```python
from build123d import *

# Parameters (mm, degrees)
MOTOR_CLAMP_EXTRUDE_DEPTH = 20
CLAMP_CLEARANCE_HOLE_D    = 3.6
CLAMP_CORNER_FILLETS_R    = 6


with BuildPart() as part:
    # Hold Down Bracket Sketch → Motor Clamp Extrude (new body)
    with BuildSketch(Plane(origin=(0, 0, 0), x_dir=(0, 0, -1), z_dir=(1, 0, 0))):
        with BuildLine():
            Line((-33.5, -23.25), (-29.5, -23.25))
            Line((-29.5, -23.25), (-29.5, -30))
            Line((-29.5, -30), (-25.5, -30))
            Line((-25.5, -30), (-25.5, -19.25))
            Line((-25.5, -19.25), (-33.5, -19.25))
            ThreePointArc((-33.5, -19.25), (-52.75, 0), (-33.5, 19.25))
            Line((-33.5, 19.25), (-25.5, 19.25))
            Line((-25.5, 19.25), (-25.5, 30))
            Line((-25.5, 30), (-29.5, 30))
            Line((-29.5, 30), (-29.5, 23.25))
            Line((-29.5, 23.25), (-33.5, 23.25))
            ThreePointArc((-33.5, 23.25), (-56.75, 0), (-33.5, -23.25))
        make_face()
    extrude(amount=MOTOR_CLAMP_EXTRUDE_DEPTH)

    # Clamp Clearance Hole (through all)
    with Locations(Plane.XY.offset(29.5)):
        with Locations((10, -26.5)):
            clamp_clearance_hole = Hole(CLAMP_CLEARANCE_HOLE_D / 2)

    # Clamp Clearance Hole Mirror: Clamp Clearance Hole across plane
    add(clamp_clearance_hole.mirror(Plane.ZX), mode=Mode.SUBTRACT)

    # Clamp Corner Fillets
    clamp_corner_fillets_edges = [part.edges().sort_by_distance(p)[0] for p in [
        (0, 30, 27.5),
        (0, -30, 27.5),
        (20, -30, 27.5),
        (20, 30, 27.5),
    ]]
    fillet(clamp_corner_fillets_edges, radius=CLAMP_CORNER_FILLETS_R)


solid = part.part
```
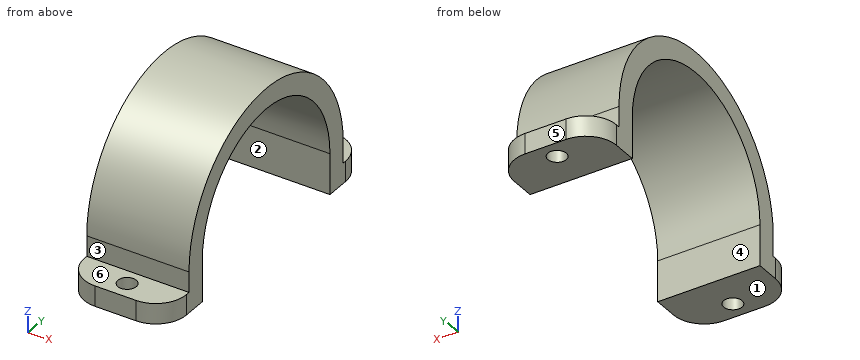
Here's how the part is built. I have some questions about the finished solid (model axes, mm). Face numbers are marked on the shaded views. A direction names the side the tool comes from. Round coordinates to 2 decimals unless told otherwise and drop trailing zeros. Write each loop counter-clockwise with the first axis right and the second up, starting at its lowest first coordinate (ties: lowest second). Pieces come first, ordered by that corner, then holes.
Q1. If we section it at B-B on y = 25.5: Write out the boundary of the cut face in (x, z), plus the area to 3 significant figures.
Q2. Which directions (+Z, -Z, +X, -X, +Y, -Y) give clear straight access to the entire face, cutting with the end or side of a thin tool? Please do the marked faces 1, 2 and 3.
Q3. If we section it at A-A on x = 10: Write out the boundary of the cut face in (y, z), plus the area to 3 significant figures.
Q4. If we section it at D-D on x = 18.5: Write out the boundary of the cut face in (y, z), plus the area to 3 significant figures.
Q5. Please list where these lines run through material, in increasing order: probe 1 along Y at (x, z) = (10, 27.2); probe 2 along Y at (x, z) = (9.5, 31); probe 3 along Y at (x, z) = (16.5, 40).
Q6. If we section it at C-C on z = 44.5: Write out the boundary of the cut face in (x, y), plus the area to 3 significant figures.
Q7. If we mould it in two halves opening along Y, with no side actions, what happens to the marked faces 4, 5 and 6? For each: +Y half, -Y half, draft (parallel to the pull), parting line (faces both ways), or undercut.
Q8. Will these pins go through, and if not, where does the flat tip stop? P1, Ø1.2, axis at x = 12.5, z = 31.5, coming from the +Y side; P2, Ø5, axis at y = -9.5, z = 45, coming from the +X side; P3, Ø12, axis at x = 9, y = -13.5, coming from the +Z side; P4, Ø3, axis at x = 11, z = 32, coming from the -Y side.
Answer below:
1. outline: (0.19, 25.5) - (8.5, 25.5) - (8.5, 29.5) - (0.19, 29.5) - close; (11.5, 25.5) - (19.81, 25.5) - (19.81, 29.5) - (11.5, 29.5) - close
1. area: 66.5 mm2
2. face 1: -Z, +X, -X, +Y, -Y
2. face 2: -Z, +X, -X
2. face 3: +Z, +X, -X, -Y
3. outline: (-30, 25.5) - (-28.3, 25.5) - (-28.3, 29.5) - (-30, 29.5) - close; (-24.7, 25.5) - (-19.25, 25.5) - (-19.25, 33.5) arc R19.25 cw to (19.25, 33.5) - (19.25, 25.5) - (24.7, 25.5) - (24.7, 29.5) - (23.25, 29.5) - (23.25, 33.5) arc R23.25 ccw to (-23.25, 33.5) - (-23.25, 29.5) - (-24.7, 29.5) - close; (28.3, 25.5) - (30, 25.5) - (30, 29.5) - (28.3, 29.5) - close
3. area: 356 mm2
4. outline: (-27.97, 25.5) - (-19.25, 25.5) - (-19.25, 33.5) arc R19.25 cw to (19.25, 33.5) - (19.25, 25.5) - (27.97, 25.5) - (27.97, 29.5) - (23.25, 29.5) - (23.25, 33.5) arc R23.25 ccw to (-23.25, 33.5) - (-23.25, 29.5) - (-27.97, 29.5) - close
4. area: 369 mm2
5. probe 1: y = -30 to -28.3, -24.7 to -19.25, 19.25 to 24.7, 28.3 to 30
5. probe 2: y = -23.25 to -19.25, 19.25 to 23.25
5. probe 3: y = -22.32 to -18.12, 18.12 to 22.32
6. outline: (0, -20.48) - (20, -20.48) - (20, -15.8) - (0, -15.8) - close; (0, 15.8) - (20, 15.8) - (20, 20.48) - (0, 20.48) - close
6. area: 187 mm2
7. face 4: undercut
7. face 5: +Y half
7. face 6: draft
8. P1: stops at y = 23.25
8. P2: passes through
8. P3: stops at z = 55.51
8. P4: stops at y = -23.25
